Can you work these out from the model? Positions are in its coordinate system, mm. A direction names the side the tool comes from. Round coordinates to 2 decimals unless told otherwise and drop trailing zeros. Order: outer loops, then holes, each group sorted by start corner. A loop starts at its lowest first (then second) coordinate and runs counter-clockwise, first axis right, second up. Notation, with made-up numbers: (1, -32) -> (58, -32) arc R12 cw to (58, -27) -> close; hole circle Ø9 at (89.5, 72). An arc over 180 degrees is marked (long way). Use a Markdown table: item, result. Add a question column.
Q1. If we section it at A-A on x = 6.5: List the corners of the cut face in (y, z) for me (3 decimals).
Q2. I need wall thicknesses on line 1 along X through (y, z) = (23, 292.1); line 2 along Z through (x, y) = (38.1, 2.5) (3 decimals); line 3 along Z through (x, y) = (12.7, 23.35). Which ranges of each line are inside material? Lowest first, please. Write a range as [from, to].
Q3. I'm going to push a flat-ended pin straight in: pin 1 Ø1.6 at (x, z) = (49.5, 328) entering from -Y. Where does the tip first touch, or does it pass through?
Q4. If we section it at C-C on z = 107: List the corners of the cut face in (x, y) for me (3 decimals), plus the area to 3 significant figures.
Q5. If we section it at B-B on y = 6.5: List the corners of the cut face in (x, z) for me (3 decimals).
Q6. For faces 1 (the face through (47.625, 13, 163)), 2 (the face through (50.8, 13, 163)), which set-ups out of +Z, -Z, +X, -X, +Y, -Y let a thin tool reach every point of the face, with its end or its side?
Q7. We'd pull the mould along Y, two halves only. Please class faces 3 (the face through (25, 25.4, 163)), 4 (the face through (25, 22.225, 163)), 5 (the face through (25, 0, 161)), 6 (the face through (27, 3, 327.025)): +Y half, -Y half, draft (parallel to the pull), parting line (faces both ways), or undercut.
```python
from build123d import *

# Parameters (mm, degrees)
SKETCH1_W           = 50.8
SKETCH1_H           = 25.4
SKETCH1_W_2         = 44.45
SKETCH1_H_2         = 19.05
BOSS_EXTRUDE1_DEPTH = 330.2
SKETCH2_W           = 50.8
SKETCH2_H           = 19.05
CUT_EXTRUDE1_DEPTH  = 3.175
SKETCH3_R           = 2.5527
CUT_EXTRUDE2_DEPTH  = 44.45


with BuildPart() as part:
    # Sketch1 → Boss-Extrude1 (new body)
    with BuildSketch(Plane.XY):
        with Locations((25.4, 12.7)):
            Rectangle(SKETCH1_W, SKETCH1_H)
        with Locations((25.4, 12.7)):
            Rectangle(SKETCH1_W_2, SKETCH1_H_2, mode=Mode.SUBTRACT)
    extrude(amount=BOSS_EXTRUDE1_DEPTH)

    # Sketch2 → Cut-Extrude1 (cut)
    with BuildSketch(Plane.XY.offset(330.2)):
        with Locations((25.4, 9.525)):
            Rectangle(SKETCH2_W, SKETCH2_H)
    extrude(amount=-CUT_EXTRUDE1_DEPTH, mode=Mode.SUBTRACT)

    # Sketch3 → Cut-Extrude2 (cut)
    with BuildSketch(Plane(origin=(0, 25.4, 0), x_dir=(1, 0, 0), z_dir=(0, 1, 0))):
        with Locations((12.7, -292.1)):
            Circle(SKETCH3_R)
        with Locations((38.1, -292.1)):
            Circle(SKETCH3_R)
        with Locations((25.4, -317.5)):
            Circle(SKETCH3_R)
    extrude(amount=-CUT_EXTRUDE2_DEPTH, mode=Mode.SUBTRACT)


solid = part.part
```
Answer below:
| question | item | result |
|---|---|---|
| 1 | outline | (0, 0) -> (3.175, 0) -> (3.175, 327.025) -> (0, 327.025) -> close; (22.225, 0) -> (25.4, 0) -> (25.4, 330.2) -> (22.225, 330.2) -> close |
| 2 | line 1 | [0, 10.15], [15.25, 35.55], [40.65, 50.8] |
| 2 | line 2 | [0, 289.547], [294.653, 327.025] |
| 2 | line 3 | [0, 289.55], [294.65, 330.2] |
| 3 | pin 1 | y = 19.05 |
| 4 | outline | (0, 0) -> (50.8, 0) -> (50.8, 25.4) -> (0, 25.4) -> close; hole (3.175, 3.175) -> (47.625, 3.175) -> (47.625, 22.225) -> (3.175, 22.225) -> close |
| 4 | area | 444 mm² |
| 5 | outline | (0, 0) -> (3.175, 0) -> (3.175, 327.025) -> (0, 327.025) -> close; (47.625, 0) -> (50.8, 0) -> (50.8, 327.025) -> (47.625, 327.025) -> close |
| 6 | face 1 | +Z, -Z |
| 6 | face 2 | +Z, -Z, +X, +Y, -Y |
| 7 | face 3 | +Y half |
| 7 | face 4 | undercut |
| 7 | face 5 | -Y half |
| 7 | face 6 | draft |
